from build123d import *

# Parameters (mm, degrees)
BOSS_EXTRUDE1_DEPTH  = 2.9
SOLENOID_PLACEMENT_W = 37.4
SOLENOID_PLACEMENT_H = 63.8
CUT_EXTRUDE1_DEPTH   = 103.571487266
CUT_EXTRUDE3_DEPTH   = 103.571487266
SKETCH4_W            = 13
SKETCH4_H            = 26.3
CUT_EXTRUDE4_DEPTH   = 98.286484159
SKETCH5_R            = 12
CUT_EXTRUDE5_DEPTH   = 98.286484159
SKETCH6_R            = 2.25
CUT_EXTRUDE6_DEPTH   = 98.286484159


with BuildPart() as part:
    # Sketch1 → Boss-Extrude1 (new body)
    with BuildSketch(Plane(origin=(0, 0, 0), x_dir=(1, 0, 0), z_dir=(0, 1, 0))):
        with BuildLine():
            ThreePointArc((33.29110537, -64.404598464), (0, 72.5), (-33.29110537, -64.404598464))
            ThreePointArc((-33.29110537, -64.404598464), (0, -44.989799638), (33.29110537, -64.404598464))
        make_face()
    extrude(amount=BOSS_EXTRUDE1_DEPTH)

    # solenoid placement → Cut-Extrude1 (cut, through all)
    with BuildSketch(Plane(origin=(0, 2.9, 0), x_dir=(1, 0, 0), z_dir=(0, 1, 0))):
        with Locations((0, -3.8)):
            Rectangle(SOLENOID_PLACEMENT_W, SOLENOID_PLACEMENT_H)
    extrude(amount=-CUT_EXTRUDE1_DEPTH, mode=Mode.SUBTRACT)

    # Sketch3 → Cut-Extrude3 (cut, through all)
    with BuildSketch(Plane(origin=(0, 2.9, 0), x_dir=(1, 0, 0), z_dir=(0, 1, 0))):
        with BuildLine():
            Line((-34.63, -32.5), (-22.83, -32.5))
            Line((-22.83, -32.5), (-22.83, 32.5))
            Line((-22.83, 32.5), (-64.807406984, 32.5))
            ThreePointArc((-64.807406984, 32.5), (-72.5, 0), (-64.807406984, -32.5))
            Line((-64.807406984, -32.5), (-34.63, -32.5))
        make_face()
        with BuildLine():
            Line((34.63, -32.5), (64.807406984, -32.5))
            ThreePointArc((64.807406984, -32.5), (72.5, 0), (64.807406984, 32.5))
            Line((64.807406984, 32.5), (22.83, 32.5))
            Line((22.83, 32.5), (22.83, -32.5))
            Line((22.83, -32.5), (34.63, -32.5))
        make_face()
    extrude(amount=-CUT_EXTRUDE3_DEPTH, mode=Mode.SUBTRACT)

    # Sketch4 → Cut-Extrude4 (cut, through all)
    with BuildSketch(Plane(origin=(0, 2.9, 0), x_dir=(1, 0, 0), z_dir=(0, 1, 0))):
        with Locations((0, 41.25)):
            Rectangle(SKETCH4_W, SKETCH4_H)
    extrude(amount=-CUT_EXTRUDE4_DEPTH, mode=Mode.SUBTRACT)

    # Sketch5 → Cut-Extrude5 (cut, through all)
    with BuildSketch(Plane(origin=(0, 2.9, 0), x_dir=(1, 0, 0), z_dir=(0, 1, 0))):
        with Locations(Location((-20, 48, 0), (0, 0, 270))):
            Circle(SKETCH5_R)
        with Locations(Location((20, 48, 0), (0, 0, 270))):
            Circle(SKETCH5_R)
    extrude(amount=-CUT_EXTRUDE5_DEPTH, mode=Mode.SUBTRACT)

    # Sketch6 → Cut-Extrude6 (cut, through all)
    with BuildSketch(Plane(origin=(0, 2.9, 0), x_dir=(1, 0, 0), z_dir=(0, 1, 0))):
        with Locations(Location((35, -50, 0), (0, 0, 270))):
            Circle(SKETCH6_R)
        with Locations(Location((-35, -50, 0), (0, 0, 270))):
            Circle(SKETCH6_R)
        with Locations(Location((-50, 40, 0), (0, 0, 270))):
            Circle(SKETCH6_R)
        with Locations(Location((50, 40, 0), (0, 0, 270))):
            Circle(SKETCH6_R)
    extrude(amount=-CUT_EXTRUDE6_DEPTH, mode=Mode.SUBTRACT)


solid = part.part
Geometry check sheet. Reference: the model listing, model coordinates, mm. A direction names the side the tool comes from. Round coordinates to 2 decimals unless told otherwise and drop trailing zeros. Write each loop counter-clockwise with the first axis right and the second up, starting at its lowest first coordinate (ties: lowest second). Pieces come first, ordered by that corner, then holes.
Item 1: Section check B-B (x = 50). Record the boundary of the cut face in (y, z), plus the area to 3 significant figures.
Determined:
outline: (0, -52.5) - (2.9, -52.5) - (2.9, -42.25) - (0, -42.25) - close; (0, -37.75) - (2.9, -37.75) - (2.9, -32.5) - (0, -32.5) - close; (0, 32.5) - (2.9, 32.5) - (2.9, 52.5) - (0, 52.5) - close
area: 103 mm2
Item 2: Material ranges on line 1 along Z through (x, y) = (13, 2.75); line 2 along X through (y, z) = (2.7, -47); line 3 along X through (y, z) = (0.5, 51), recorded low to high.
Determined:
line 1: z = -71.32 to -57.75, -38.25 to -28.1, 35.7 to 47.27
line 2: x = -55.2 to -31.96, -8.04 to -6.5, 6.5 to 8.04, 31.96 to 55.2
line 3: x = -51.53 to -37.02, -32.98 to -20.58, 20.58 to 32.98, 37.02 to 51.53
Item 3: Access from +Z, -Z, +X, -X, +Y, -Y to the whole of each face (thin tool, end or side, straight path). Record for faces 1 (the face through (44, 1, -32.5)), 2 (the face through (-13, 1, -28.1)), 3 (the face through (-44, 1, -32.5)), 4 (the face through (51.35, 1.43, 51.18)).
Determined:
face 1: +X, +Y, -Y
face 2: +Y, -Y
face 3: -X, +Y, -Y
face 4: +Z, +X, +Y, -Y
Item 4: Go/stop test with flat-tipped pins: pin 1 Ø0.9 at (x, y) = (5, 2) entering from -Z; pin 2 Ø1.4 at (x, y) = (-42, 1) entering from -Z; pin 3 Ø0.9 at (x, y) = (-53.5, 1) entering from +Z. Record where each tip stops, or that it passes through.
Determined:
pin 1: stops at z = -72.36
pin 2: stops at z = -59.59
pin 3: stops at z = 49.42
Item 5: Section check C-C (y = 0.45). Record the boundary of the cut face in (x, z).
Determined:
outline: (-64.81, -32.5) arc R72.5 ccw to (64.81, -32.5) - (22.83, -32.5) - (22.83, 32.5) - (64.81, 32.5) arc R72.5 ccw to (33.29, 64.4) arc R38.25 cw to (-33.29, 64.4) arc R72.5 ccw to (-64.81, 32.5) - (-22.83, 32.5) - (-22.83, -32.5) - close; hole circle Ø4.5 at (-50, -40); hole circle Ø4.5 at (-35, 50); hole circle Ø24 at (-20, -48); hole (-18.7, -28.1) - (-6.5, -28.1) - (-6.5, -54.4) - (6.5, -54.4) - (6.5, -28.1) - (18.7, -28.1) - (18.7, 35.7) - (-18.7, 35.7) - close; hole circle Ø24 at (20, -48); hole circle Ø4.5 at (35, 50); hole circle Ø4.5 at (50, -40)
Item 6: Section check A-A (z = 29). Record the boundary of the cut face in (x, y), plus the area to 3 significant figures.
Determined:
outline: (-22.83, 0) - (-18.7, 0) - (-18.7, 2.9) - (-22.83, 2.9) - close; (18.7, 0) - (22.83, 0) - (22.83, 2.9) - (18.7, 2.9) - close
area: 24.0 mm2
Item 7: Mould release check, pull along Z, two halves, no side actions. Record for faces 5 (the face through (19, 0, -4)), 6 (the face through (-33.48, 1.47, 48.34)), 7 (the face through (-0.565, 1.43, 44.994)): +Z half, -Z half, draft (parallel to the pull), parting line (faces both ways), or undercut.
Determined:
face 5: draft
face 6: undercut
face 7: +Z half
Item 8: Section check D-D (z = -40). Record the boundary of the cut face in (x, y).
Determined:
outline: (-60.47, 0) - (-52.25, 0) - (-52.25, 2.9) - (-60.47, 2.9) - close; (-47.75, 0) - (-28.94, 0) - (-28.94, 2.9) - (-47.75, 2.9) - close; (-11.06, 0) - (-6.5, 0) - (-6.5, 2.9) - (-11.06, 2.9) - close; (6.5, 0) - (11.06, 0) - (11.06, 2.9) - (6.5, 2.9) - close; (28.94, 0) - (47.75, 0) - (47.75, 2.9) - (28.94, 2.9) - close; (52.25, 0) - (60.47, 0) - (60.47, 2.9) - (52.25, 2.9) - close
